from build123d import *

# Parameters (mm, degrees)
BOSS_EXTRUDE1_DEPTH = 2
SKETCH3_W           = 3
SKETCH3_H           = 11
CUT_EXTRUDE1_DEPTH  = 2
CHAMFER1_SIZE       = 2
SKETCH4_W           = 9
SKETCH4_H           = 22
CUT_EXTRUDE2_DEPTH  = 2


with BuildPart() as part:
    # Sketch1 → Boss-Extrude1 (new body)
    with BuildSketch(Plane(origin=(0, 0, 0), x_dir=(1, 0, 0), z_dir=(0, 1, 0))):
        with BuildLine():
            Line((-29.25, -24.848942598), (28.75, -24.848942598))
            ThreePointArc((28.75, -24.848942598), (30.164213562, -24.263156161), (30.75, -22.848942598))
            Line((30.75, -22.848942598), (30.75, 10.651057402))
            ThreePointArc((30.75, 10.651057402), (30.164213562, 12.065270964), (28.75, 12.651057402))
            Line((28.75, 12.651057402), (-29.25, 12.651057402))
            ThreePointArc((-29.25, 12.651057402), (-30.664213562, 12.065270964), (-31.25, 10.651057402))
            Line((-31.25, 10.651057402), (-31.25, -22.848942598))
            ThreePointArc((-31.25, -22.848942598), (-30.664213562, -24.263156161), (-29.25, -24.848942598))
        make_face()
    extrude(amount=BOSS_EXTRUDE1_DEPTH)

    # Sketch3 → Cut-Extrude1 (cut)
    with BuildSketch(Plane(origin=(0, 2, 0), x_dir=(1, 0, 0), z_dir=(0, 1, 0))):
        with Locations((-29.75, -5.848942598)):
            Rectangle(SKETCH3_W, SKETCH3_H)
    extrude(amount=-CUT_EXTRUDE1_DEPTH, mode=Mode.SUBTRACT)

    # Chamfer1
    chamfer1_edges = [part.edges().sort_by_distance(p)[0] for p in [
        (-31.25, 1, 11.348942598),
        (-31.25, 1, 0.348942598),
    ]]
    chamfer(chamfer1_edges, length=CHAMFER1_SIZE)

    # Sketch4 → Cut-Extrude2 (cut)
    with BuildSketch(Plane(origin=(0, 2, 0), x_dir=(1, 0, 0), z_dir=(0, 1, 0))):
        with Locations((26.25, -5.848942598)):
            Rectangle(SKETCH4_W, SKETCH4_H)
    extrude(amount=-CUT_EXTRUDE2_DEPTH, mode=Mode.SUBTRACT)


solid = part.part
Build history of the part. All positions in model axes, mm. A direction names the side the tool comes from. Give positions to 0.01 mm unless a question says otherwise; leave off trailing zeros. Order: outer loops, then holes, each group sorted by start corner. A loop starts at its lowest first (then second) coordinate and runs counter-clockwise, first axis right, second up. Notation, with made-up numbers: M -16.75,27.5 L -1.75,27.5 A8 ccw -1.75,39.5 Z; hole C -28.5,56 d11. An arc over 180 degrees is marked long. Use one line per item in the form item = value.
Q1. Slice it at C-C, the plane z = 15. Write the cut outline in (x, y), and give its area (3 significant figures).
Conclusion:
outline = M -31.25,0 L 21.75,0 L 21.75,2 L -31.25,2 Z
area = 106 mm2
Q2. Which spindle directions (+Z, -Z, +X, -X, +Y, -Y) get a long thin tool onto all of the face, cutting with end or side? Do faces 1 (the flat face through (26, 1, 16.849)), 2 (the flat face through (-30.3, 1, -0.7)), 3 (the flat face through (0, 1, -12.651)). Say none if no direction does.
Conclusion:
face_1 = +X, +Y, -Y
face_2 = -X, +Y, -Y
face_3 = -Z, +X, -X, +Y, -Y
Q3. Slice it at B-B, the plane y = 1.15. Write the cut outline in (x, z).
Conclusion:
outline = M -31.25,-10.65 A2 ccw -29.25,-12.65 L 28.75,-12.65 A2 ccw 30.75,-10.65 L 30.75,-5.15 L 21.75,-5.15 L 21.75,16.85 L 30.75,16.85 L 30.75,22.85 A2 ccw 28.75,24.85 L -29.25,24.85 A2 ccw -31.25,22.85 L -31.25,13.35 L -29.25,11.35 L -28.25,11.35 L -28.25,0.35 L -29.25,0.35 L -31.25,-1.65 Z
Q4. Pull direction Z, two halves, no side cores. Call faces 4 (the cylindrical face through (-30.65, 0.99, -12.08)), 5 (the flat face through (30.75, 1, -8)), 6 (the flat face through (-30.2, 1, 12.3)): released by +Z, released by -Z, zero draft, split by the parting line, or undercut.
Conclusion:
face_4 = released by -Z
face_5 = zero draft
face_6 = undercut
Q5. Wall check: probe 1 along Z at (x, y) = (23.5, 1.2); probe 2 along X at (y, z) = (1.65, 4.5); probe 3 along X at (y, z) = (0.5, 16.5). Give the ranges that are in metal, low to high.
Conclusion:
probe_1 = -12.65 to -5.15, 16.85 to 24.85
probe_2 = -28.25 to 21.75
probe_3 = -31.25 to 21.75
Q6. Pin check, flat tip, straight feed: P1, Ø1, axis at y = 0.5, z = 10.5, coming from the +X side. Stop position of the tip, or through.
Conclusion:
P1 = 21.75
Q7. Slice it at D-D, the plane z = 5. Write the cut outline in (x, y), and give its area (3 significant figures).
Conclusion:
outline = M -28.25,0 L 21.75,0 L 21.75,2 L -28.25,2 Z
area = 100 mm2
Q8. Slice it at A-A, the plane x = 27. Write the cut outline in (y, z), and give its area (3 significant figures).
Conclusion:
outline = M 0,-12.65 L 2,-12.65 L 2,-5.15 L 0,-5.15 Z; M 0,16.85 L 2,16.85 L 2,24.85 L 0,24.85 Z
area = 31.0 mm2
